from build123d import *

# Parameters (mm, degrees)
SKETCH1_R             = 2.5
BOSS_EXTRUDE1_DEPTH   = 10
BOSS_EXTRUDE1_2_DEPTH = 10
BOSS_EXTRUDE2_DEPTH   = 3
SKETCH3_R             = 0.8125
CUT_EXTRUDE1_DEPTH    = 18
CHAMFER1_SIZE         = 0.8
SKETCH4_R             = 1.6
CUT_EXTRUDE2_DEPTH    = 10


with BuildPart() as part:
    # Sketch1 → Boss-Extrude1 (new body)
    with BuildSketch(Plane(origin=(0, 0, 0), x_dir=(0, 1, 0), z_dir=(0, 0, 1))):
        with Locations((-35, 0)):
            Circle(SKETCH1_R)
    extrude(amount=BOSS_EXTRUDE1_DEPTH)



with BuildPart() as body_2:
    # Sketch1 → Boss-Extrude1 2 (new body)
    with BuildSketch(Plane(origin=(0, 0, 0), x_dir=(0, 1, 0), z_dir=(0, 0, 1))):
        with Locations((35, 0)):
            Circle(SKETCH1_R)
    extrude(amount=BOSS_EXTRUDE1_2_DEPTH)


with BuildPart() as part_1:
    add(part.part)

    add(body_2.part)  # Boss-Extrude2 merges body 2
    # Sketch2 → Boss-Extrude2 (add)
    with BuildSketch(Plane(origin=(0, 0, 0), x_dir=(1, 0, 0), z_dir=(0, 0, -1))):
        with BuildLine():
            Line((6.5, 35), (6.5, -35))
            ThreePointArc((6.5, -35), (0, -41.5), (-6.5, -35))
            Line((-6.5, -35), (-6.5, 35))
            ThreePointArc((-6.5, 35), (0, 41.5), (6.5, 35))
        make_face()
    extrude(amount=BOSS_EXTRUDE2_DEPTH)

    # Sketch3 → Cut-Extrude1 (cut)
    with BuildSketch(Plane.XY.offset(10)):
        with Locations((0, -35)):
            Circle(SKETCH3_R)
        with Locations((0, 35)):
            Circle(SKETCH3_R)
    extrude(amount=-CUT_EXTRUDE1_DEPTH, mode=Mode.SUBTRACT)

    # Chamfer1
    chamfer1_edges = [part_1.edges().sort_by_distance(p)[0] for p in [
        (0, 32.5, 0),
        (0, -37.5, 0),
    ]]
    chamfer(chamfer1_edges, length=CHAMFER1_SIZE)

    # Sketch4 → Cut-Extrude2 (cut)
    with BuildSketch(Plane.XY):
        with Locations((0, 22.5)):
            Circle(SKETCH4_R)
        with Locations(Location((0, -22.5, 0), (0, 0, 180))):
            Circle(SKETCH4_R)
    extrude(amount=-CUT_EXTRUDE2_DEPTH, mode=Mode.SUBTRACT)


solid = part_1.part
The listing builds one solid part. Answer for the finished solid, in the listing's coordinates (mm). A direction names the side the tool comes from. Give positions to 0.01 mm unless a question says otherwise; leave off trailing zeros. Loops run counter-clockwise (first coordinate to the right, second up) from the corner with the lowest first, then second, coordinate; pieces in that order, holes last. Notation, with made-up numbers: M 5.25,8.5 L 51.25,8.5 A25 cw 51.25,44.5 Z; hole C 20.5,61 d11. An arc over 180 degrees is marked long. Answer as CSV lines item,"result".
Item 1: The part is cut by section C-C (z = 3). Give the vertices of the cut face in (x, y) (1 decimal).
Values follow:
outline,"C 0,-35 d5; C 0,35 d5; hole C 0,-35 d1.6; hole C 0,35 d1.6"
Item 2: The part is cut by section B-B (x = 0). Give the number of separate pieces and of enclosed holes in the cut face, and give its area (3 significant figures).
Values follow:
separate pieces,"5"
enclosed holes,"0"
area,"289 mm^2"
Item 3: The mould has two halves that part along X. Classify faces 3 (the flat face through (6.5, 0, -1)), 4 (the cylindrical face through (0.96, 37.31, 5.34)), 5 (the flat face through (0, -1, 0)), 6 (the cylindrical face through (0.375, -35.721, 3.591)): released by +X, released by -X, zero draft, split by the parting line, or undercut.
Values follow:
face 3,"released by +X"
face 4,"split by the parting line"
face 5,"zero draft"
face 6,"undercut"
Item 4: Straight lines are drawn through the part: line 1 along Y through (x, z) = (0, -1.25); line 2 along Y through (x, z) = (0, 4.25); line 3 along X through (y, z) = (35, 4.75). For each, find the intervals that lie inside material, in ascending order. Write a range as [from, to].
Values follow:
line 1,"y = [-41.5, -35.81], [-34.19, -24.1], [-20.9, 20.9], [24.1, 34.19], [35.81, 41.5]"
line 2,"y = [-37.5, -35.81], [-34.19, -32.5], [32.5, 34.19], [35.81, 37.5]"
line 3,"x = [-2.5, -0.81], [0.81, 2.5]"
Item 5: Which of the six approach directions +Z, -Z, +X, -X, +Y, -Y give full straight-line access (tool end or side, diameter ignored) to faces 1 (the cylindrical face through (0.1, 41.5, -1.5)), 2 (the cylindrical face through (0.96, -32.69, 5.34))?
Values follow:
face 1,"+Z, -Z, +Y"
face 2,"+Z"
Item 6: Given pin 1 Ø4 at (x, y) = (-1.5, -13.5) entering from +Z; pin 2 Ø3 at (x, z) = (0, 3) entering from -Y; pin 3 Ø3 at (x, z) = (0, 2.5) entering from +Y, each flat-ended and moving along its own axis, determine where each tip first touches the part or whether it passes through.
Values follow:
pin 1,"stops at z = 0"
pin 2,"stops at y = -37.5"
pin 3,"stops at y = 37.5"
Item 7: The part is cut by section A-A (y = 22.5). Give the vertices of the cut face in (x, z).
Values follow:
outline,"M -6.5,-3 L -1.6,-3 L -1.6,0 L -6.5,0 Z; M 1.6,-3 L 6.5,-3 L 6.5,0 L 1.6,0 Z"
Item 8: The part is cut by section D-D (y = 1.5). Give the vertices of the cut face in (x, z).
Values follow:
outline,"M -6.5,-3 L 6.5,-3 L 6.5,0 L -6.5,0 Z"
